Could you check a few things on this model? Use its own coordinates, in mm. A direction names the side the tool comes from. Give positions to 0.01 mm unless a question says otherwise; leave off trailing zeros. Loops run counter-clockwise (first coordinate to the right, second up) from the corner with the lowest first, then second, coordinate; pieces in that order, holes last. Notation, with made-up numbers: M 66,50.25 L 98,50.25 A9 ccw 98,63.25 Z; hole C -27,-35.5 d10. An arc over 180 degrees is marked long. Use CSV: the item, a comma, the result in double quotes.
```python
from build123d import *

# Parameters (mm, degrees)
SKETCH1_W           = 50.8
SKETCH1_H           = 50.8
BOSS_EXTRUDE1_DEPTH = 50.8
SKETCH2_R           = 12.7
BOSS_EXTRUDE2_DEPTH = 25.4
SKETCH3_R           = 12.7
CUT_EXTRUDE1_DEPTH  = 25.4


with BuildPart() as part:
    # Sketch1 → Boss-Extrude1 (new body)
    with BuildSketch(Plane.XY):
        Rectangle(SKETCH1_W, SKETCH1_H)
    extrude(amount=BOSS_EXTRUDE1_DEPTH)

    # Sketch2 → Boss-Extrude2 (add)
    with BuildSketch(Plane.XY.offset(50.8)):
        with Locations(Location((0, 0, 0), (0, 0, 180))):
            Circle(SKETCH2_R)
    extrude(amount=BOSS_EXTRUDE2_DEPTH)

    # Sketch3 → Cut-Extrude1 (cut)
    with BuildSketch(Plane(origin=(0, 0, 0), x_dir=(-1, 0, 0), z_dir=(0, 0, -1))):
        Circle(SKETCH3_R)
    extrude(amount=-CUT_EXTRUDE1_DEPTH, mode=Mode.SUBTRACT)


solid = part.part
```
1. I want a section at A-A, the plane z = 17. List the corners of the cut face in (x, y) for me, then the cut area to 3 significant figures.
Outcome:
outline,"M -25.4,-25.4 L 25.4,-25.4 L 25.4,25.4 L -25.4,25.4 Z; hole C 0,0 d25.4"
area,"2,070 mm2"
2. I'm going to push flat-ended pins straight in: pin 1 Ø10 at (x, z) = (-4, 61.5) entering from -Y; pin 2 Ø23 at (x, y) = (0, 0) entering from -Z. Where does each tip first touch, or does it pass through?
Outcome:
pin 1,"y = -12.7"
pin 2,"z = 25.4"
3. If we mould it in two halves opening along Y, with no side actions, what happens to faces 4 (the face through (0, -25.4, 25)), 5 (the face through (0, 0, 25.4)), 6 (the face through (0, 25.4, 25)), 7 (the face through (25.4, 0, 25))? For each: +Y half, -Y half, draft (parallel to the pull), parting line (faces both ways), or undercut.
Outcome:
face 4,"-Y half"
face 5,"undercut"
face 6,"+Y half"
face 7,"draft"
4. I want a section at C-C, the plane x = -15. List the corners of the cut face in (y, z) for me.
Outcome:
outline,"M -25.4,0 L 25.4,0 L 25.4,50.8 L -25.4,50.8 Z"
5. Please list where these lines run through material, in increasing order: line 1 (Y direction, x = 0, z = 12.5); line 2 (Z direction, x = -1.5, y = 7); line 3 (Z direction, x = 22, y = 16.5).
Outcome:
line 1,"-25.4 to -12.7, 12.7 to 25.4"
line 2,"25.4 to 76.2"
line 3,"0 to 50.8"
6. I want a section at B-B, the plane y = 0. List the corners of the cut face in (x, z) for me, then the cut area to 3 significant figures.
Outcome:
outline,"M -25.4,0 L -12.7,0 L -12.7,25.4 L 12.7,25.4 L 12.7,0 L 25.4,0 L 25.4,50.8 L 12.7,50.8 L 12.7,76.2 L -12.7,76.2 L -12.7,50.8 L -25.4,50.8 Z"
area,"2,580 mm2"
7. Which directions (+Z, -Z, +X, -X, +Y, -Y) give clear straight access to the entire face, cutting with the end or side of a thin tool? Please do faces 1 (the face through (-6, 12, 0)), 2 (the face through (2.75, -12.4, 12.52)), 3 (the face through (-5.86, 11.267, 63.322)).
Outcome:
face 1,"-Z, +X, -X, +Y, -Y"
face 2,"-Z"
face 3,"+Z"
